CAD build for the part. Positions are in the model's coordinates, mm. Give positions to 0.01 mm unless a question says otherwise; leave off trailing zeros. Order: outer loops, then holes, each group sorted by start corner. A loop starts at its lowest first (then second) coordinate and runs counter-clockwise, first axis right, second up.
from build123d import *

# Parameters (mm, degrees)
ESQUISSE1_W               = 120
ESQUISSE1_H               = 40
T_LE_DE_BASE_PLI_E1_DEPTH = 6
D_GAGEMENT_M61_D          = 7


# Sheet-metal steps are written as plain solids
with BuildPart() as part:
    # Esquisse1 → Tôle de base pliée1 (new body)
    with BuildSketch(Plane(origin=(0, 0, 0), x_dir=(1, 0, 0), z_dir=(0, 1, 0))):
        Rectangle(ESQUISSE1_W, ESQUISSE1_H)
    extrude(amount=-T_LE_DE_BASE_PLI_E1_DEPTH)

    # Dégagement M61 (through all)
    with Locations(Plane(origin=(0, 0, 0), x_dir=(1, 0, 0), z_dir=(0, 1, 0))):
        with Locations((54, 0), (-54, 0)):
            Hole(D_GAGEMENT_M61_D / 2)


solid = part.part
1. Saw through at C-C on y = -3.75. Give the cut face in (x, z).
2. Mould opens along X. For faces 1 (the cylindrical face through (-50.503, -3.042, -0.154)), 2 (the flat face through (-1, -3, -20)), 3 (the flat face through (60, -3, 0)), 4 (the flat face through (-60, -3, 0)) say: released by +X, released by -X, zero draft, split by the parting line, or undercut.
3. Saw through at A-A on x = -54. Give the cut face in (y, z), plus the area to 3 significant figures.
4. Wall check: line 1 (Z direction, x = -54, y = -1.25); line 2 (Z direction, x = 51, y = -5). Give the ranges that are in metal, low to high.
5. Saw through at B-B on z = 0. Give the cut face in (x, y).
Reported:
1. outline: (-60, -20) - (60, -20) - (60, 20) - (-60, 20) - close; hole circle Ø7 at (-54, 0); hole circle Ø7 at (54, 0)
2. face 1: undercut
2. face 2: zero draft
2. face 3: released by +X
2. face 4: released by -X
3. outline: (-6, -20) - (0, -20) - (0, -3.5) - (-6, -3.5) - close; (-6, 3.5) - (0, 3.5) - (0, 20) - (-6, 20) - close
3. area: 198 mm2
4. line 1: z = -20 to -3.5, 3.5 to 20
4. line 2: z = -20 to -1.8, 1.8 to 20
5. outline: (-60, -6) - (-57.5, -6) - (-57.5, 0) - (-60, 0) - close; (-50.5, -6) - (50.5, -6) - (50.5, 0) - (-50.5, 0) - close; (57.5, -6) - (60, -6) - (60, 0) - (57.5, 0) - close
